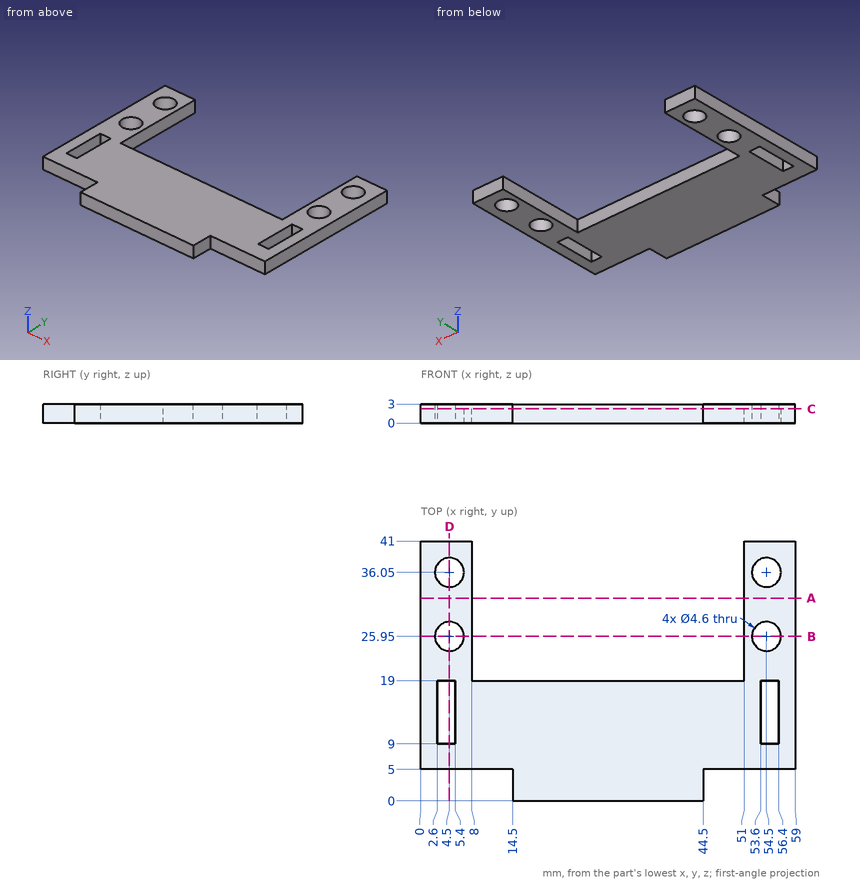
Job drawing, mm, ordinate dimensions from the low corner. One solid piece. Round coordinates to 2 decimals unless told otherwise and drop trailing zeros. Loops run counter-clockwise (first coordinate to the right, second up) from the corner with the lowest first, then second, coordinate; pieces in that order, holes last. Notation, with made-up numbers: M 59,-9.5 L 73,-9.5 A5 cw 73,-5.5 Z; hole C -4,-11.5 d8. An arc over 180 degrees is marked long. Answer as CSV lines item,"result".
1. Cut at B-B on y = 25.95. Write the cut outline in (x, z), then the cut area to 3 significant figures.
Resolved:
outline,"M 0,0 L 2.2,0 L 2.2,3 L 0,3 Z; M 6.8,0 L 8,0 L 8,3 L 6.8,3 Z; M 51,0 L 52.2,0 L 52.2,3 L 51,3 Z; M 56.8,0 L 59,0 L 59,3 L 56.8,3 Z"
area,"20.4 mm²"
2. Wall check: probe 1 along Y at (x, z) = (54.5, 1.35); probe 2 along X at (y, z) = (17, 0.95); probe 3 along X at (y, z) = (33.5, 1.95). Give the ranges that are in metal, low to high. Write a range as [from, to].
Resolved:
probe 1,"y = [5, 9], [19, 23.65], [28.25, 33.75], [38.35, 41]"
probe 2,"x = [0, 2.6], [5.4, 53.6], [56.4, 59]"
probe 3,"x = [0, 8], [51, 59]"
3. Flat gauge pin, fed straight in: P1, Ø0.9, axis at x = 50, z = 2, coming from the -Y side. Where does the tip first touch, or does it go through?
Resolved:
P1,"stops at y = 5"
4. Cut at C-C on z = 2.25. Write the cut outline in (x, y).
Resolved:
outline,"M 0,5 L 14.5,5 L 14.5,0 L 44.5,0 L 44.5,5 L 59,5 L 59,41 L 51,41 L 51,19 L 8,19 L 8,41 L 0,41 Z; hole C 4.5,25.95 d4.6; hole C 4.5,36.05 d4.6; hole M 2.6,9 L 5.4,9 L 5.4,19 L 2.6,19 Z; hole C 54.5,25.95 d4.6; hole C 54.5,36.05 d4.6; hole M 53.6,9 L 56.4,9 L 56.4,19 L 53.6,19 Z"
5. Cut at A-A on y = 32. Write the cut outline in (x, z).
Resolved:
outline,"M 0,0 L 8,0 L 8,3 L 0,3 Z; M 51,0 L 59,0 L 59,3 L 51,3 Z"
6. Cut at D-D on x = 4.5. Write the cut outline in (y, z), then the cut area to 3 significant figures.
Resolved:
outline,"M 5,0 L 9,0 L 9,3 L 5,3 Z; M 19,0 L 23.65,0 L 23.65,3 L 19,3 Z; M 28.25,0 L 33.75,0 L 33.75,3 L 28.25,3 Z; M 38.35,0 L 41,0 L 41,3 L 38.35,3 Z"
area,"50.4 mm²"
